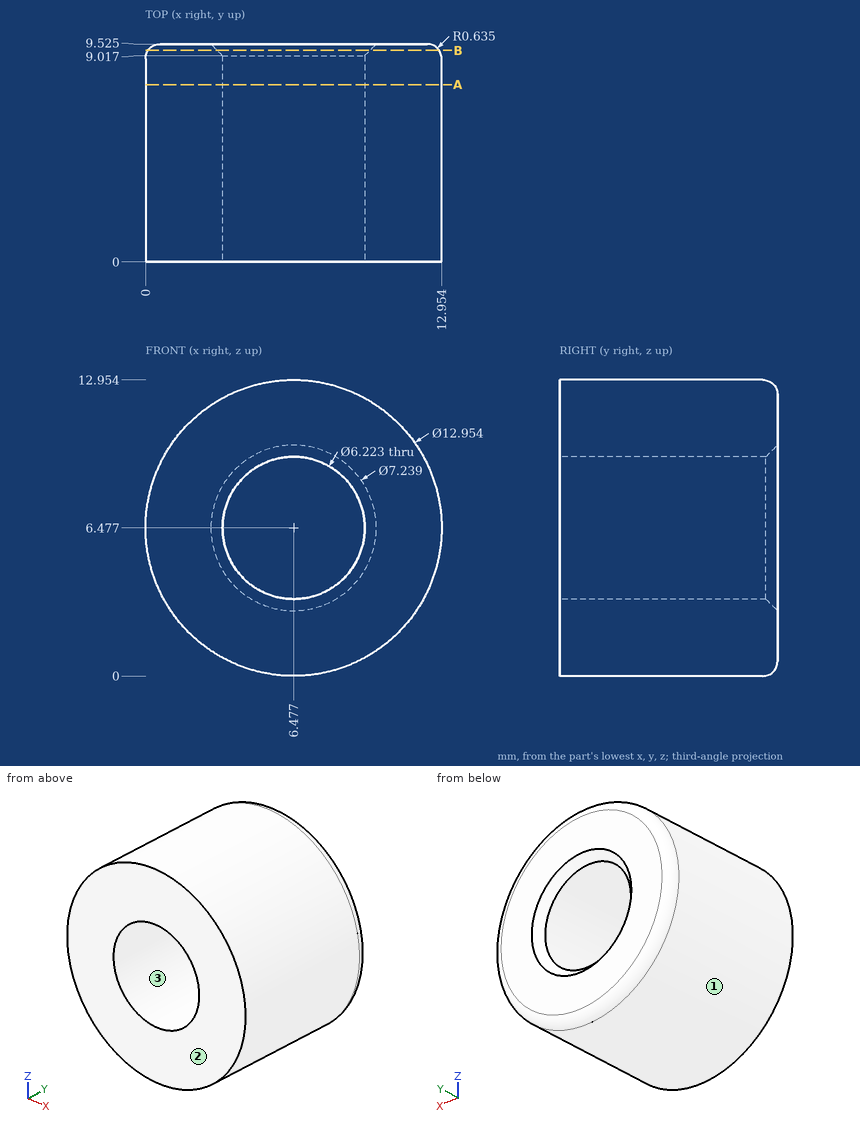
Geometry check sheet. Reference: drawing and pictorial views, mm from the part's lowest x, y, z. Round coordinates to 2 decimals unless told otherwise and drop trailing zeros. Loops run counter-clockwise (first coordinate to the right, second up) from the corner with the lowest first, then second, coordinate; pieces in that order, holes last. Notation, with made-up numbers: (13, 27.25) - (38, 27.25) arc R20 ccw to (38, 34.25) - close; hole circle Ø10 at (70, 86.5). An arc over 180 degrees is marked (long way). One line per question, with ' | ' between items. Start each with the question number.
1. Cross-section at B-B on y = 9.25. Record the cut outline in (x, z), then the cut area to 3 significant figures.
2. Scan lines: line 1 (Z direction, x = 6.5, y = 1); line 2 (Z direction, x = 7, y = 2.25); line 3 (X direction, y = 6, z = 8.5). Record each from-to range of solid material in increasing order. Write a range as [from, to].
3. Draft check along X on the marked faces 1, 2 and 3. Enter one of: released by +X, released by -X, zero draft, split by the parting line, or undercut.
4. Cross-section at A-A on y = 7.75. Record the cut outline in (x, z).
5. Depth check by flat-ended pin: pin 1 (3 mm diameter, centred on x = 1.5, y = 4, fed in from +Z); pin 2 (4 mm diameter, centred on x = 11.5, y = 1.5, fed in from -Z); pin 3 (4 mm diameter, centred on y = 4, z = 1.5, fed in from -X). Enter the tip coordinate at first touch or a pass-through.
Taken from the geometry:
1) outline: circle Ø12.73 at (6.48, 6.48); hole circle Ø6.69 at (6.48, 6.48) | area: 92.1 mm²
2) line 1: [0, 3.37], [9.59, 12.95] | line 2: [0.02, 3.41], [9.54, 12.93] | line 3: [0.32, 4.11], [8.84, 12.63]
3) face 1: split by the parting line | face 2: zero draft | face 3: undercut
4) outline: circle Ø12.95 at (6.48, 6.48); hole circle Ø6.22 at (6.48, 6.48)
5) pin 1: z = 11.94 | pin 2: z = 0.75 | pin 3: x = 0.72
